Build history of the part. All positions in model axes, mm. A direction names the side the tool comes from. Coordinates: 2 decimals unless noted, no trailing zeros. Write each loop counter-clockwise with the first axis right and the second up, starting at its lowest first coordinate (ties: lowest second). Pieces come first, ordered by that corner, then holes. Notation, with made-up numbers: (-37.5, -3) -> (-23.5, -3) arc R8 ccw to (-23.5, 5) -> close; hole circle Ø3 at (-13, -16.5). An arc over 180 degrees is marked (long way). Write each question's results on one line, items separated by ' | '. Start each with the question number.
Q1. Two-plate mould, pull along Y, no slides. Class faces 1 (the face through (2.54, -23, 20)), 2 (the face through (25, -25, 0)), 3 (the face through (25, -48.26, 20)), 4 (the face through (25, 0, 19)): released by +Y, released by -Y, zero draft, split by the parting line, or undercut.
Q2. Drop a flat-ended pin along its axis: pin 1 Ø13.5 at (x, y) = (36, -32) entering from +Z. Give the stop position or say it passes through.
Q3. Tool access for faces 5 (the face through (25, -25, 2.54)), 6 (the face through (23, -50, 38.1)): list every direction of +Z, -Z, +X, -X, +Y, -Y with a clear straight run to the whole face (end or side of a thin tool).
Q4. Saw through at B-B on z = 14. Give the cut face in (x, y), and give its area (3 significant figures).
Q5. Saw through at A-A on x = 20. Give the cut face in (y, z), and give its area (3 significant figures).
Q6. Drill centre lines: line 1 (X direction, y = -25.5, z = 34.5); line 2 (Y direction, x = 40.5, z = 27); line 3 (Z direction, x = 38.5, y = -12). Where is each one in solid material? Low to high.
Q7. Saw through at C-C on y = -27.5. Give the cut face in (x, z), and give its area (3 significant figures).
from build123d import *

# Parameters (mm, degrees)
F0_W     = 50.8
F0_H     = 50.8
F1_DEPTH = 38.1
F2_R     = 7.62
F3_T     = -2.54


with BuildPart() as f1:
    # F0 (on Top) → F1 (new body)
    with BuildSketch(Plane.XY):
        with Locations((25.4, -25.4)):
            Rectangle(F0_W, F0_H)
    extrude(amount=F1_DEPTH)

    # F2
    f2_edges = [f1.edges().sort_by_distance(p)[0] for p in [
        (50.8, -50.8, 19.05),
        (0, -50.8, 19.05),
    ]]
    fillet(f2_edges, radius=F2_R)

    # F3
    f3_openings = [f1.faces().sort_by_distance(p)[0] for p in [
        (25.4, -25.168915, 38.1),
    ]]
    offset(amount=F3_T, openings=f3_openings)


solid = f1.part
Returned:
1) face 1: undercut | face 2: zero draft | face 3: undercut | face 4: released by +Y
2) pin 1: stops at z = 2.54
3) face 5: +Z | face 6: +Z, +X, -X, +Y, -Y
4) outline: (0, -43.18) arc R7.62 ccw to (7.62, -50.8) -> (43.18, -50.8) arc R7.62 ccw to (50.8, -43.18) -> (50.8, 0) -> (0, 0) -> close; hole (2.54, -43.18) arc R5.08 ccw to (7.62, -48.26) -> (43.18, -48.26) arc R5.08 ccw to (48.26, -43.18) -> (48.26, -2.54) -> (2.54, -2.54) -> close | area: 476 mm2
5) outline: (-50.8, 0) -> (0, 0) -> (0, 38.1) -> (-2.54, 38.1) -> (-2.54, 2.54) -> (-48.26, 2.54) -> (-48.26, 38.1) -> (-50.8, 38.1) -> close | area: 310 mm2
6) line 1: x = 0 to 2.54, 48.26 to 50.8 | line 2: y = -50.8 to -48.26, -2.54 to 0 | line 3: z = 0 to 2.54
7) outline: (0, 0) -> (50.8, 0) -> (50.8, 38.1) -> (48.26, 38.1) -> (48.26, 2.54) -> (2.54, 2.54) -> (2.54, 38.1) -> (0, 38.1) -> close | area: 310 mm2
